from build123d import *

# Parameters (mm, degrees)
SKETCH_1_W                = 90
SKETCH_1_H                = 40
EXTRUDE_1_DEPTH           = 8
SKETCH_2_R                = 1.5
CUT_EXTRUDE_1_DEPTH       = 50.889878733
SKETCH_3_W                = 90
SKETCH_3_H                = 8
EXTRUDE_2_DEPTH           = 35
CUT_EXTRUDE_3_DEPTH       = 61.415229868
SKETCH_7_W                = 22
SKETCH_7_H                = 40
CUT_EXTRUDE_4_DEPTH       = 66.375836515
SKETCH_8_W                = 5
SKETCH_8_H                = 32
EXTRUDE_3_DEPTH           = 35
CUT_EXTRUDE_5_DEPTH       = 59.576872569
SKETCH_14_R               = 1.5
CUT_EXTRUDE_8_DEPTH       = 70.641941386
SKETCH_15_W               = 12
SKETCH_15_H               = 11
CUT_EXTRUDE_10_DEPTH      = 70.641941386
FILLET_2_R                = 5
FILLET_5_R                = 5
CUT_EXTRUDE_11_DEPTH      = 66.375836515
CUT_EXTRUDE_11_DEPTH_BACK = 66.375836515
FILLET_4_R                = 10
CUT_EXTRUDE_12_DEPTH      = 66.375836515
SKETCH_19_W               = 6
SKETCH_19_H               = 20
EXTRUDE_4_DEPTH           = 20
CUT_EXTRUDE_13_REACH      = 67.008
FILLET_6_R                = 3


with BuildPart() as part:
    # 草图1 → 凸台-拉伸1 (new body)
    with BuildSketch(Plane(origin=(0, 0, 0), x_dir=(1, 0, 0), z_dir=(0, 1, 0))):
        Rectangle(SKETCH_1_W, SKETCH_1_H)
    extrude(amount=EXTRUDE_1_DEPTH)

    # 草图2 → 切除-拉伸1 (cut, through all)
    with BuildSketch(Plane.XZ):
        with Locations(Location((-14, -4.5, 0), (0, 0, 270))):
            Circle(SKETCH_2_R)
        with Locations(Location((-14, -15.5, 0), (0, 0, 270))):
            Circle(SKETCH_2_R)
        with Locations(Location((14, -15.5, 0), (0, 0, 90))):
            Circle(SKETCH_2_R)
        with Locations(Location((14, -4.5, 0), (0, 0, 90))):
            Circle(SKETCH_2_R)
    extrude(amount=-CUT_EXTRUDE_1_DEPTH, mode=Mode.SUBTRACT)

    # 草图3 → 凸台-拉伸2 (add)
    with BuildSketch(Plane.XZ):
        with Locations((0, 16)):
            Rectangle(SKETCH_3_W, SKETCH_3_H)
    extrude(amount=EXTRUDE_2_DEPTH)

    # 草图6 → 切除-拉伸3 (cut, through all)
    with BuildSketch(Plane.XZ):
        Polygon((-45, 12), (-20, -20), (-45, -20), align=None)
    extrude(amount=-CUT_EXTRUDE_3_DEPTH, mode=Mode.SUBTRACT)

    # 草图7 → 切除-拉伸4 (cut, through all)
    with BuildSketch(Plane(origin=(0, 8, 0), x_dir=(1, 0, 0), z_dir=(0, 1, 0))):
        with Locations((34, 0)):
            Rectangle(SKETCH_7_W, SKETCH_7_H)
    extrude(amount=-CUT_EXTRUDE_4_DEPTH, mode=Mode.SUBTRACT)

    # 草图8 → 凸台-拉伸3 (add)
    with BuildSketch(Plane.XZ):
        with Locations((0, -4)):
            Rectangle(SKETCH_8_W, SKETCH_8_H)
    extrude(amount=EXTRUDE_3_DEPTH)

    # 草图9 → 切除-拉伸5 (cut, through all)
    with BuildSketch(Plane.ZY.offset(2.5)):
        Polygon((-20, 0), (12, -35), (-20, -35), align=None)
    extrude(amount=-CUT_EXTRUDE_5_DEPTH, mode=Mode.SUBTRACT)

    # 草图14 → 切除-拉伸8 (cut, through all)
    with BuildSketch(Plane.XY.offset(20)):
        with Locations((-8.576116211, -24.051679616)):
            Circle(SKETCH_14_R)
        with Locations((-38.352500761, -27.707759918)):
            Circle(SKETCH_14_R)
        with Locations((-40.789887629, -7.856836885)):
            Circle(SKETCH_14_R)
        with Locations((-11.013503079, -4.200756583)):
            Circle(SKETCH_14_R)
    extrude(amount=-CUT_EXTRUDE_8_DEPTH, mode=Mode.SUBTRACT)

    # 草图15 → 切除-拉伸10 (cut, through all)
    with BuildSketch(Plane.XY.offset(20)):
        with Locations((-24, -29.5)):
            Rectangle(SKETCH_15_W, SKETCH_15_H)
    extrude(amount=-CUT_EXTRUDE_10_DEPTH, mode=Mode.SUBTRACT)

    # 圆角2
    fillet_2_edges = [part.edges().sort_by_distance(p)[0] for p in [
        (-30, -24, 16),
        (-18, -24, 16),
    ]]
    fillet(fillet_2_edges, radius=FILLET_2_R)

    # 圆角5
    fillet_5_edges = [part.edges().sort_by_distance(p)[0] for p in [
        (2.5, 0, -4),
        (-2.5, 0, -4),
    ]]
    fillet(fillet_5_edges, radius=FILLET_5_R)

    # 草图16 → 切除-拉伸11 (cut, two sides: drawn at the far end of the back side and taken through both)
    with BuildSketch(Plane(origin=(0, 0, 12), x_dir=(-1, 0, 0), z_dir=(0, 0, -1)).offset(-CUT_EXTRUDE_11_DEPTH_BACK)):
        Polygon((-23, 0), (-2.5, -35), (-23, -35), align=None)
    extrude(amount=CUT_EXTRUDE_11_DEPTH + CUT_EXTRUDE_11_DEPTH_BACK, mode=Mode.SUBTRACT)

    # 圆角4
    fillet_4_edges = [part.edges().sort_by_distance(p)[0] for p in [
        (-45, -35, 16),
        (-20, 4, -20),
        (23, 4, -20),
    ]]
    fillet(fillet_4_edges, radius=FILLET_4_R)

    # 草图18 → 切除-拉伸12 (cut, through all)
    with BuildSketch(Plane(origin=(0, 8, 0), x_dir=(1, 0, 0), z_dir=(0, 1, 0))):
        with BuildLine():
            Line((11, -12), (11, -20))
            Line((11, -20), (23, -20))
            Line((23, -20), (23, -12))
            Line((23, -12), (23, 0))
            ThreePointArc((23, 0), (14.514718626, -3.514718626), (11, -12))
        make_face()
    extrude(amount=-CUT_EXTRUDE_12_DEPTH, mode=Mode.SUBTRACT)

    # 草图19 → 凸台-拉伸4 (add)
    with BuildSketch(Plane(origin=(0, 0, 12), x_dir=(-1, 0, 0), z_dir=(0, 0, -1))):
        with Locations((25, -10)):
            Rectangle(SKETCH_19_W, SKETCH_19_H)
    extrude(amount=EXTRUDE_4_DEPTH)

    # 草图20 → 切除-拉伸13 (cut, up to next)
    with BuildSketch(Plane.ZY.offset(28), mode=Mode.PRIVATE) as cut_extrude_13_sk1:
        Polygon((-8, 0), (12, -20), (-8, -20), align=None)
    cut_extrude_13_tool1 = extrude(cut_extrude_13_sk1.sketch, amount=-CUT_EXTRUDE_13_REACH, mode=Mode.PRIVATE) & part.part
    add(cut_extrude_13_tool1.solids().sort_by_distance((-28, -13.333333, -1.333333))[0], mode=Mode.SUBTRACT)

    # 圆角6
    # the kernel refuses this fillet: 3 mm, written as the material it adds along each edge
    with BuildSketch(Plane(origin=(-22, 0, 19.5), x_dir=(1, 0, 0), z_dir=(0, 0, -1))) as fillet_6_piece_1_section:
        with BuildLine():
            CenterArc((FILLET_6_R, FILLET_6_R), FILLET_6_R, 180, 90)
            Line((0, FILLET_6_R), (0, 0))
            Line((0, 0), (FILLET_6_R, 0))
        make_face()
    fillet_6_piece_1 = extrude(amount=35, mode=Mode.PRIVATE)
    fillet_6_piece_1 = split(fillet_6_piece_1, bisect_by=Plane(origin=(-21.320814657, -12.214592671, 4.214592671), z_dir=(0, 0.7071067811865476, 0.7071067811865476)), keep=Keep.TOP, mode=Mode.PRIVATE)
    add(fillet_6_piece_1)
    with BuildSketch(Plane(origin=(-28, 0, 19.5), x_dir=(-1, 0, 0), z_dir=(0, 0, -1))) as fillet_6_piece_2_section:
        with BuildLine():
            CenterArc((FILLET_6_R, -FILLET_6_R), FILLET_6_R, 90, 90)
            Line((0, -FILLET_6_R), (0, 0))
            Line((0, 0), (FILLET_6_R, 0))
        make_face()
    fillet_6_piece_2 = extrude(amount=35, mode=Mode.PRIVATE)
    fillet_6_piece_2 = split(fillet_6_piece_2, bisect_by=Plane(origin=(-28.679185343, -12.214592671, 4.214592671), z_dir=(0, 0.7071067811865476, 0.7071067811865476)), keep=Keep.TOP, mode=Mode.PRIVATE)
    fillet_6_piece_2 = split(fillet_6_piece_2, bisect_by=Plane(origin=(-40.633408635, -0.679185343, 6.410763053), z_dir=(0.7880243737245634, 0, 0.6156440419723153)), keep=Keep.TOP, mode=Mode.PRIVATE)
    add(fillet_6_piece_2)


solid = part.part
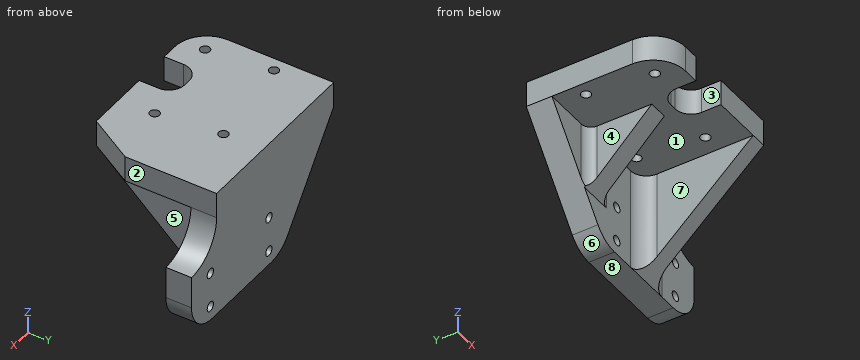
Design review of the part built by this model. Coordinates are the model's own, in mm. Face numbers are marked on the shaded views. A direction names the side the tool comes from. Give positions to 0.01 mm unless a question says otherwise; leave off trailing zeros. Loops run counter-clockwise (first coordinate to the right, second up) from the corner with the lowest first, then second, coordinate; pieces in that order, holes last. Notation, with made-up numbers: (-12, 80) - (39, 80) arc R14 cw to (39, 92) - close; hole circle Ø1 at (10.25, -13). An arc over 180 degrees is marked (long way). Write item = value, one per line.
1) Clearance check with flat-ended pins moving along their axes: pin 1 Ø5 at (x, z) = (-27.5, 7.5) entering from -Y; pin 2 Ø3.5 at (x, z) = (14, -4.5) entering from -Y; pin 3 Ø2.5 at (x, y) = (7, -23.5) entering from -Z; pin 4 Ø3.5 at (x, y) = (-38.35, -27.71) entering from +Z. State where each tip first meets the part, or that it passes through.
Result sheet:
pin_1 = -18
pin_2 = 0
pin_3 = 12
pin_4 = 20
2) Draft analysis for pull direction X (two halves, no side actions). For the marked faces 6, 7 and 8, state which applies: +X half, -X half, draft (parallel to the pull), parting line (faces both ways), or undercut.
Result sheet:
face_6 = -X half
face_7 = undercut
face_8 = draft
3) Take a section at B-B on y = 2. State the section outline as (x, z) points, and give its area (3 significant figures).
Result sheet:
outline = (-45, 12) - (-23, -16.16) arc R10 ccw to (-15.12, -20) - (13, -20) arc R10 ccw to (23, -10) - (23, 0) arc R12 cw to (11, 12) - (11, 20) - (-45, 20) - close; hole circle Ø3 at (-14, -15.5); hole circle Ø3 at (-14, -4.5); hole circle Ø3 at (14, -15.5); hole circle Ø3 at (14, -4.5)
area = 2,060 mm2
4) Take a section at C-C on x = 14. State the section outline as (y, z) points, and give its area (3 significant figures).
Result sheet:
outline = (0, -19.95) - (8, -19.95) - (8, -17) - (0, -17) - close; (0, -14) - (8, -14) - (8, -6) - (0, -6) - close; (0, -3) - (8, -3) - (8, 4.06) - (0, 4.06) - close
area = 144 mm2
5) Tool access review of the marked faces 1, 2, 3, 4 and 5: name each direction out of +Z, -Z, +X, -X, +Y, -Y from which nothing blocks a thin tool from reaching the whole face with its end or side.
Result sheet:
face_1 = -Z, -Y
face_2 = +Z, +X, +Y, -Y
face_3 = +Z, -Z, -Y
face_4 = -Z, -X, -Y
face_5 = -Z, +X, -Y
6) To check wall thickness, follow line 1 (X direction, y = 1, z = -15); line 2 (Z direction, x = 14, y = 2.5); line 3 (X direction, y = 4, z = -4.5). State the ranges of each line that lie inside material, in increasing order.
Result sheet:
line_1 = -23.91 to -15.41, -12.59 to 12.59, 15.41 to 21.66
line_2 = -19.95 to -17, -14 to -6, -3 to 4.06
line_3 = -32.11 to -15.5, -12.5 to 12.5, 15.5 to 23
7) Take a section at A-A on x = -14. State the section outline as (y, z) points, and give its area (3 significant figures).
Result sheet:
outline = (-35, 12) - (0, 12) - (0, -3) - (8, -3) - (8, 20) - (-35, 20) - close; (0, -20) - (8, -20) - (8, -17) - (0, -17) - close; (0, -14) - (8, -14) - (8, -6) - (0, -6) - close
area = 552 mm2
